The model under review builds one solid part; all positions refer to its coordinate system, in mm. Face numbers are marked on the shaded views. Round coordinates to 2 decimals unless told otherwise and drop trailing zeros. Write each loop counter-clockwise with the first axis right and the second up, starting at its lowest first coordinate (ties: lowest second). Pieces come first, ordered by that corner, then holes. Notation, with made-up numbers: M 25.25,65.5 L 78.25,65.5 A32 cw 78.25,101.5 Z; hole C 39,75.25 d4. An arc over 180 degrees is marked long. Write item = value, one per line. Start each with the question number.
Item 1: Take a section at C-C, the plane y = 16. Give the boundary of the cut face in (x, z).
Item 2: Take a section at B-B, the plane x = 0. Give the boundary of the cut face in (y, z).
Item 3: To check wall thickness, follow line 1 along Y through (x, z) = (28.8, 0); line 2 along X through (y, z) = (12.75, 0); line 3 along Z through (x, y) = (2, 4.75). State the ranges of each line that lie inside material, in increasing order.
Item 4: The part is to be moulded in two halves that separate along X. For the marked faces 1, 2 and 3, say which applies: +X half, -X half, draft (parallel to the pull), parting line (faces both ways), or undercut.
Item 5: Take a section at A-A, the plane z = 0. Give the boundary of the cut face in (x, y), plus the area to 3 significant figures.
Item 6: For pin 1 Ø8 at (y, z) = (4, 18) entering from -X; pin 2 Ø3 at (x, y) = (18, 4) entering from -Z; pin 3 Ø4 at (y, z) = (11, 18) entering from +X, all flat-tipped, find the tip position at first contact; note any pin that passes through.
Item 7: Take a section at D-D, the plane z = 16. Give the boundary of the cut face in (x, y).
from build123d import *

# Parameters (mm, degrees)
SKETCH1_R               = 27.686
BOSS_EXTRUDE1_DEPTH     = 19.05
CUT_EXTRUDE1_REACH      = 72.221
CUT_EXTRUDE1_END_RADIUS = 27.686
SKETCH2_R               = 2.667
CIRPATTERN1_COUNT       = 8


with BuildPart() as part:
    # Sketch1 → Boss-Extrude1 (new body)
    with BuildSketch(Plane(origin=(0, 0, 0), x_dir=(1, 0, 0), z_dir=(0, 1, 0))):
        Polygon((12.520019136, 30.226), (-12.520019136, 30.226), (-30.226, 12.520019136), (-30.226, -12.520019136), (-12.520019136, -30.226), (12.520019136, -30.226), (30.226, -12.520019136), (30.226, 12.520019136), align=None)
        with Locations(Location((0, 0, 0), (0, 0, 90))):
            Circle(SKETCH1_R, mode=Mode.SUBTRACT)
    extrude(amount=BOSS_EXTRUDE1_DEPTH)

    # Cut-Extrude1: up to this cylinder (the profile starts outside it)
    cut_extrude1_end = Plane(origin=(0, 9.525, 0), z_dir=(0, -1, 0)) * Cylinder(CUT_EXTRUDE1_END_RADIUS, 200.814, mode=Mode.PRIVATE)
    # Sketch2 → Cut-Extrude1 (cut, up to the surface)
    with BuildSketch(Plane.XY.offset(30.226), mode=Mode.PRIVATE) as cut_extrude1_sk1:
        with Locations((0, 9.525)):
            Circle(SKETCH2_R)
    cut_extrude1_tool1 = extrude(cut_extrude1_sk1.sketch, amount=-CUT_EXTRUDE1_REACH, mode=Mode.PRIVATE) - cut_extrude1_end
    cut_extrude1 = cut_extrude1_tool1.solids().sort_by_distance((0, 9.525, 30.226))[0]
    add(cut_extrude1, mode=Mode.SUBTRACT)

    # CirPattern1: Cut-Extrude1 ×8 about axis
    cirpattern1_axis = Axis((0, 19.05, 0), (0, 1, 0))
    for i in range(1, CIRPATTERN1_COUNT):
        add(cut_extrude1.rotate(cirpattern1_axis, i * 360 / CIRPATTERN1_COUNT), mode=Mode.SUBTRACT)


solid = part.part
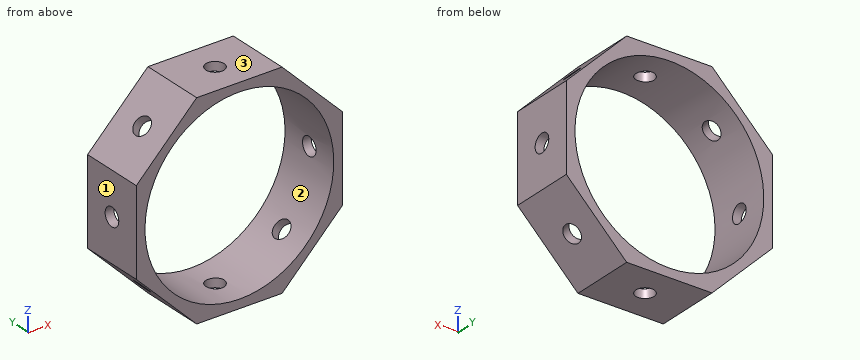
Response values:
q1.outline = M -30.23,-12.52 L -12.52,-30.23 L 12.52,-30.23 L 30.23,-12.52 L 30.23,12.52 L 12.52,30.23 L -12.52,30.23 L -30.23,12.52 Z; hole C 0,0 d55.37
q2.outline = M 0,-30.23 L 6.86,-30.23 L 6.86,-27.69 L 0,-27.69 Z; M 0,27.69 L 6.86,27.69 L 6.86,30.23 L 0,30.23 Z; M 12.19,-30.23 L 19.05,-30.23 L 19.05,-27.69 L 12.19,-27.69 Z; M 12.19,27.69 L 19.05,27.69 L 19.05,30.23 L 12.19,30.23 Z
q3.line_1 = 0 to 6.86, 12.19 to 19.05
q3.line_2 = -30.23 to -27.69, 27.69 to 30.23
q3.line_3 = -30.23 to -27.61, 27.61 to 30.23
q4.face_1 = -X half
q4.face_2 = undercut
q4.face_3 = draft
q5.outline = M -30.23,0 L -27.69,0 L -27.69,6.86 L -30.23,6.86 Z; M -30.23,12.19 L -27.69,12.19 L -27.69,19.05 L -30.23,19.05 Z; M 27.69,0 L 30.23,0 L 30.23,6.86 L 27.69,6.86 Z; M 27.69,12.19 L 30.23,12.19 L 30.23,19.05 L 27.69,19.05 Z
q5.area = 69.7 mm2
q6.pin_1 = -28.75
q6.pin_2 = -26.25
q6.pin_3 = 26.75
q7.outline = M -26.75,0 L -22.59,0 L -22.59,19.05 L -26.75,19.05 Z; M 22.59,0 L 26.75,0 L 26.75,19.05 L 22.59,19.05 Z
